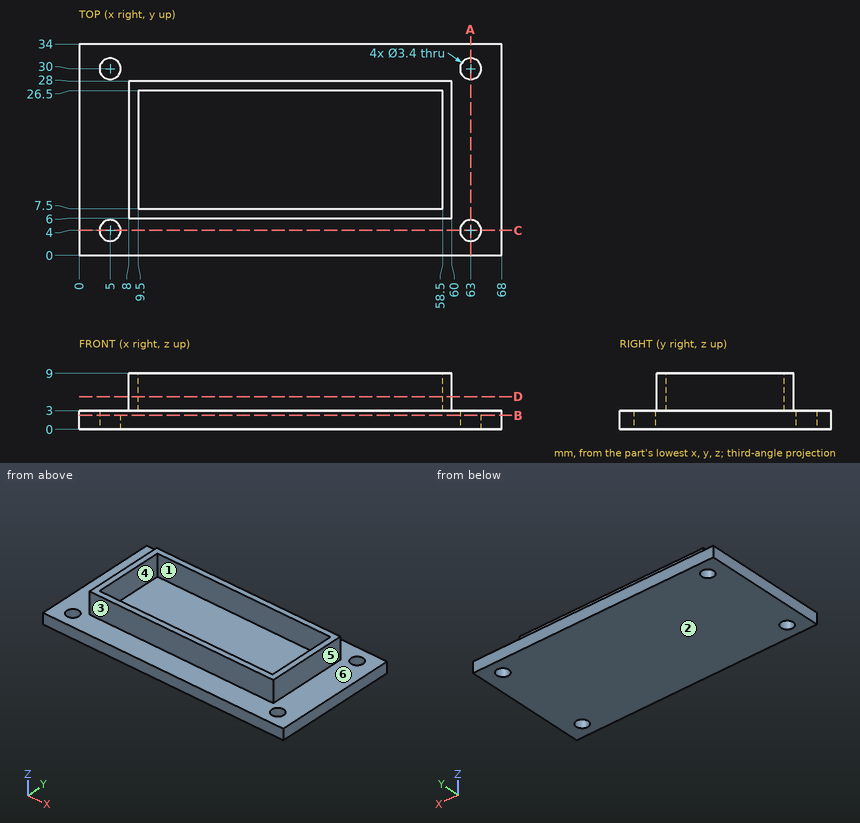
Check sheet for the drawn part. Datum: minimum x, y, z corner. Units: mm. A direction names the side the tool comes from. Round coordinates to 2 decimals unless told otherwise and drop trailing zeros. Loops run counter-clockwise (first coordinate to the right, second up) from the corner with the lowest first, then second, coordinate; pieces in that order, holes last. Notation, with made-up numbers: (36.25, 74.25) - (79.25, 74.25) arc R21 cw to (79.25, 112.25) - close; hole circle Ø8 at (34, 55). An arc over 180 degrees is marked (long way). Answer as a JSON object with one key per item and string values. Group by question number.
Q1. Set-up check for the marked faces 1, 2 and 3: record each of +Z, -Z, +X, -X, +Y, -Y from which the full face is reachable in a straight line by a thin tool's end or side.
Q2. Sectioned sample at C-C, the plane y = 4. Enter the section's corners in (x, z).
Q3. Mould release check, pull along X, two halves, no side actions. Record for the marked faces 4, 5 and 6: released by +X, released by -X, zero draft, split by the parting line, or undercut.
Q4. Scan lines: line 1 along Y through (x, z) = (5, 1); line 2 along X through (y, z) = (16.5, 7.5); line 3 along Y through (x, z) = (26, 3.25). Record each from-to range of solid material in increasing order. Write a range as [from, to].
Q5. Gauge pin test, flat ends, axial feed: P1, Ø5, axis at x = 57, y = 22, coming from the -Z side; P2, Ø1.8, axis at x = 42, z = 7, coming from the -Y side; P3, Ø10, axis at x = 26, y = 15.5, coming from the +Z side; P4, Ø2.5, axis at x = 63, y = 30, coming from the +Z side. Record the tip position at first contact, or that the pin passes through.
Q6. Sectioned sample at D-D, the plane z = 5.25. Enter the section's corners in (x, y), plus the area to 3 significant figures.
Q7. Sectioned sample at B-B, the plane z = 2.25. Enter the section's corners in (x, y), plus the area to 3 significant figures.
Q8. Sectioned sample at A-A, the plane x = 63. Enter the section's corners in (y, z).
Solution:
{
 "1": {"face 1": "+Z", "face 2": "-Z, +X, -X, +Y, -Y", "face 3": "+Z, +X, -X, -Y"},
 "2": {"outline": "(0, 0) - (3.3, 0) - (3.3, 3) - (0, 3) - close; (6.7, 0) - (61.3, 0) - (61.3, 3) - (6.7, 3) - close; (64.7, 0) - (68, 0) - (68, 3) - (64.7, 3) - close"},
 "3": {"face 4": "undercut", "face 5": "released by +X", "face 6": "zero draft"},
 "4": {"line 1": "y = [0, 2.3], [5.7, 28.3], [31.7, 34]", "line 2": "x = [8, 9.5], [58.5, 60]", "line 3": "y = [6, 7.5], [26.5, 28]"},
 "5": {"P1": "stops at z = 0", "P2": "stops at y = 6", "P3": "stops at z = 3", "P4": "passes through"},
 "6": {"outline": "(8, 6) - (60, 6) - (60, 28) - (8, 28) - close; hole (9.5, 7.5) - (58.5, 7.5) - (58.5, 26.5) - (9.5, 26.5) - close", "area": "213 mm²"},
 "7": {"outline": "(0, 0) - (68, 0) - (68, 34) - (0, 34) - close; hole circle Ø3.4 at (5, 4); hole circle Ø3.4 at (5, 30); hole circle Ø3.4 at (63, 4); hole circle Ø3.4 at (63, 30)", "area": "2,280 mm²"},
 "8": {"outline": "(0, 0) - (2.3, 0) - (2.3, 3) - (0, 3) - close; (5.7, 0) - (28.3, 0) - (28.3, 3) - (5.7, 3) - close; (31.7, 0) - (34, 0) - (34, 3) - (31.7, 3) - close"}
}
